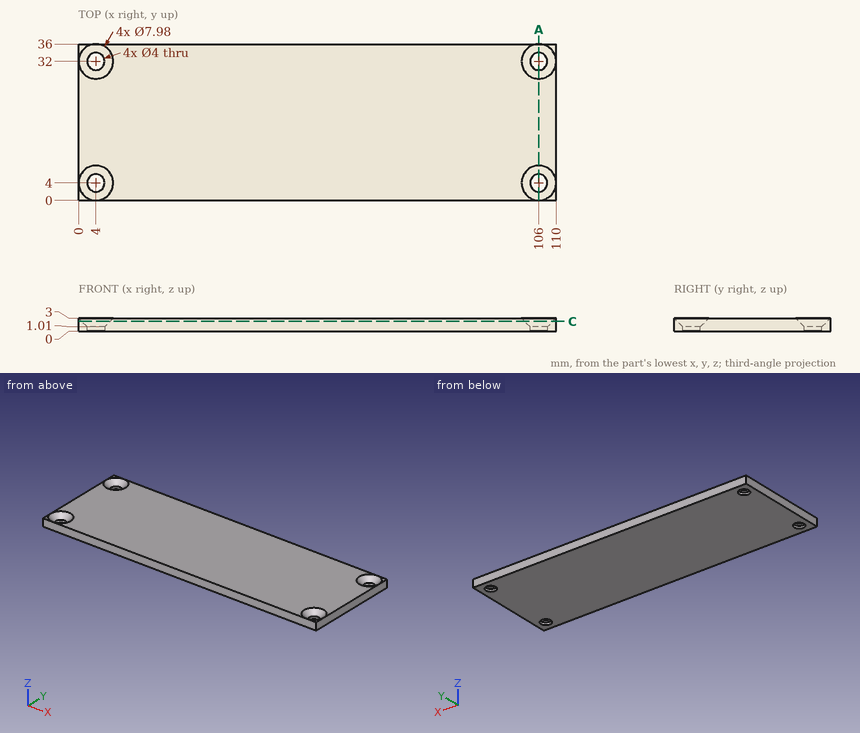
Answer from the drawing. Dimensions are ordinates in mm from the lowest x, y and z of the part. Round coordinates to 2 decimals unless told otherwise and drop trailing zeros. Write each loop counter-clockwise with the first axis right and the second up, starting at its lowest first coordinate (ties: lowest second). Pieces come first, ordered by that corner, then holes. Notation, with made-up numbers: (14.5, 24.25) - (53.5, 24.25) arc R26 ccw to (53.5, 38.25) - close; hole circle Ø3 at (68, 50). An arc over 180 degrees is marked (long way). Use a Markdown table: item, result.
(1) The part is cut by section C-C (z = 2.3). Write down the section's boundary in (x, y).
Reported:
| item | result |
|---|---|
| outline | (0, 0) - (110, 0) - (110, 36) - (0, 36) - close; hole circle Ø6.58 at (4, 4); hole circle Ø6.58 at (4, 32); hole circle Ø6.58 at (106, 4); hole circle Ø6.58 at (106, 32) |
(2) Straight lines are drawn through the part: line 1 along Y through (x, z) = (4, 0.7); line 2 along X through (y, z) = (31, 2.1); line 3 along X through (y, z) = (31, 0.6). For each, find the intervals that lie inside material, in ascending order. Write a range as [from, to].
Reported:
| item | result |
|---|---|
| line 1 | [0, 2], [6, 30], [34, 36] |
| line 2 | [0, 1.08], [6.92, 103.08], [108.92, 110] |
| line 3 | [0, 2.27], [5.73, 104.27], [107.73, 110] |
(3) The part is cut by section A-A (x = 106). State how many separate pieces and enclosed holes the cut face has, then the cut area to 3 significant figures.
Reported:
| item | result |
|---|---|
| separate pieces | 3 |
| enclosed holes | 0 |
| area | 76.1 mm2 |
